from build123d import *

# Parameters (mm, degrees)
F0_R          = 56.8109783896
F1_DEPTH      = 12.7
F2_R          = 50.5287562703
F3_DEPTH      = 177.8
F4_R          = 35.56
F5_DEPTH      = 203.2
F6_W          = 133.571790182
F6_H          = 62.377858907
F7_DEPTH      = 203.2
F7_DEPTH_BACK = 25.4


with BuildPart() as f1:
    # F0 (on Top) → F1 (new body)
    with BuildSketch(Plane.XY):
        Circle(F0_R)
    extrude(amount=F1_DEPTH)

    # F2 (on face) → F3 (join)
    with BuildSketch(Plane(origin=(0, 0, 0), x_dir=(1, 0, 0), z_dir=(0, 0, -1))):
        Circle(F2_R)
    extrude(amount=F3_DEPTH)

    # F4 (on face) → F5 (cut)
    with BuildSketch(Plane.XY.offset(12.7)):
        Circle(F4_R)
    extrude(amount=-F5_DEPTH, mode=Mode.SUBTRACT)

    # F6 (on Top) → F7 (cut, two sides)
    with BuildSketch(Plane.XY) as f7_sk:
        with Locations((2.2456042352, -31.1889294535)):
            Rectangle(F6_W, F6_H)
    extrude(amount=-F7_DEPTH, mode=Mode.SUBTRACT)
    extrude(f7_sk.sketch, amount=F7_DEPTH_BACK, mode=Mode.SUBTRACT)


solid = f1.part
The model under review builds one solid part; all positions refer to its coordinate system, in mm. A direction names the side the tool comes from. Give positions to 0.01 mm unless a question says otherwise; leave off trailing zeros. Order: outer loops, then holes, each group sorted by start corner. A loop starts at its lowest first (then second) coordinate and runs counter-clockwise, first axis right, second up. Notation, with made-up numbers: M -37,9 L 18,9 A23 cw 18,47 Z; hole C 70,68 d3. An arc over 180 degrees is marked long. Use one line per item in the form item = value. Start each with the question number.
Item 1: We need section A-A on y = 15.5. Give the boundary of the cut face in (x, z).
Item 2: We need section D-D on y = 5. Give the boundary of the cut face in (x, z), plus the area to 3 significant figures.
Item 3: We need section C-C on z = -4. Give the boundary of the cut face in (x, y).
Item 4: To check wall thickness, follow line 1 along Z through (x, y) = (-19.5, 49.5); line 2 along X through (y, z) = (26, -68); line 3 along Y through (x, z) = (-0.5, -167). State the ranges of each line that lie inside material, in increasing order. Write a range as from..to.
Item 5: For faces 1 (the flat face through (-1, 41, 12.7)), 2 (the flat face through (0, 52, 0)), list the 3-axis set-ups (+Z, -Z, +X, -X, +Y, -Y) from which the entire face can be reached by the end or side of a thin tool; tool diameter is ignored.
Item 6: Insertion check: pin 1 Ø1 at (y, z) = (36.5, -144.5) entering from -X; pin 2 Ø4 at (y, z) = (13.5, -90) entering from -X; pin 3 Ø10 at (y, z) = (31.5, -132.5) entering from +X. Each pin has a flat end and moves straight along its axis. Give the tip position at first contact, or say it passes through.
Item 7: We need section B-B on x = 0. Give the boundary of the cut face in (y, z).
Completed:
q1.outline = M -54.66,0 L -48.09,0 L -48.09,-177.8 L -32,-177.8 L -32,12.7 L -54.66,12.7 Z; M 32,-177.8 L 48.09,-177.8 L 48.09,0 L 54.66,0 L 54.66,12.7 L 32,12.7 Z
q2.outline = M -56.59,0 L -50.28,0 L -50.28,-177.8 L -35.21,-177.8 L -35.21,12.7 L -56.59,12.7 Z; M 35.21,-177.8 L 50.28,-177.8 L 50.28,0 L 56.59,0 L 56.59,12.7 L 35.21,12.7 Z
q2.area = 5,900 mm²
q3.outline = M -50.53,0 L -35.56,0 A35.56 cw 35.56,0 L 50.53,0 A50.53 ccw Z
q4.line_1 = 0..12.7
q4.line_2 = -43.33..-24.26, 24.26..43.33
q4.line_3 = 35.56..50.53
q5.face_1 = +Z, +X, -X, +Y, -Y
q5.face_2 = -Z, +Y
q6.pin_1 = -35.46
q6.pin_2 = -49.2
q6.pin_3 = 43.02
q7.outline = M 35.56,-177.8 L 50.53,-177.8 L 50.53,0 L 56.81,0 L 56.81,12.7 L 35.56,12.7 Z
